For this review, take the finished solid that the model builds, in its own axes (mm). A direction names the side the tool comes from. Coordinates: 2 decimals unless noted, no trailing zeros. Loops run counter-clockwise (first coordinate to the right, second up) from the corner with the lowest first, then second, coordinate; pieces in that order, holes last. Notation, with made-up numbers: M -3,53.5 L 12,53.5 A30 ccw 12,77.5 Z; hole C 76.5,22 d4. An arc over 180 degrees is marked long. Use one line per item in the form item = value.
```python
from build123d import *

# Parameters (mm, degrees)
SKETCH1_W           = 69.85
SKETCH1_H           = 38.1
BOSS_EXTRUDE1_DEPTH = 3.175
SKETCH2_W           = 3.175
SKETCH2_H           = 3.175
BOSS_EXTRUDE2_DEPTH = 3.175
SKETCH3_W           = 20.32
SKETCH3_H           = 3.175
BOSS_EXTRUDE3_DEPTH = 3.175


with BuildPart() as part:
    # Sketch1 → Boss-Extrude1 (new body)
    with BuildSketch(Plane.XY):
        Rectangle(SKETCH1_W, SKETCH1_H)
    extrude(amount=BOSS_EXTRUDE1_DEPTH)

    # Sketch2 → Boss-Extrude2 (add)
    with BuildSketch(Plane(origin=(0, 0, 0), x_dir=(-1, 0, 0), z_dir=(0, 0, -1))):
        with Locations((-36.5125, 17.4625)):
            Rectangle(SKETCH2_W, SKETCH2_H)
        with Locations((-36.5125, -4.7625)):
            Rectangle(SKETCH2_W, SKETCH2_H)
        with Locations((36.5125, 17.4625)):
            Rectangle(SKETCH2_W, SKETCH2_H)
        with Locations((36.5125, -4.7625)):
            Rectangle(SKETCH2_W, SKETCH2_H)
    extrude(amount=-BOSS_EXTRUDE2_DEPTH)

    # Sketch3 → Boss-Extrude3 (add)
    with BuildSketch(Plane.XZ.offset(19.05)):
        with Locations((-16.51, 1.5875)):
            Rectangle(SKETCH3_W, SKETCH3_H)
        with Locations((16.51, 1.5875)):
            Rectangle(SKETCH3_W, SKETCH3_H)
    extrude(amount=BOSS_EXTRUDE3_DEPTH)


solid = part.part
```
1. Consider section C-C on x = 0. Write out the cut boundary in (y, z) (3 decimals).
Computed values:
outline = M -19.05,0 L 19.05,0 L 19.05,3.175 L -19.05,3.175 Z
2. Wall thickness on line 1 along X through (y, z) = (-20, 2.15); line 2 along X through (y, z) = (-13.5, 1.1) (3 decimals); line 3 along Y through (x, z) = (29, 1.95): over which ranges is each line inside the solid? List them lowest first. Write a range as from..to.
Computed values:
line_1 = -26.67..-6.35, 6.35..26.67
line_2 = -34.925..34.925
line_3 = -19.05..19.05
3. Draft analysis for pull direction Y (two halves, no side actions). For faces 6 (the face through (-36, -6.35, 2)), 7 (the face through (-38.1, -5, 2)), 8 (the face through (-36, 15.875, 2)), state which applies: +Y half, -Y half, draft (parallel to the pull), parting line (faces both ways), or undercut.
Computed values:
face_6 = -Y half
face_7 = draft
face_8 = undercut
4. Consider section A-A on z = 2.4. Write out the cut boundary in (x, y) (3 decimals).
Computed values:
outline = M -38.1,-6.35 L -34.925,-6.35 L -34.925,-19.05 L -26.67,-19.05 L -26.67,-22.225 L -6.35,-22.225 L -6.35,-19.05 L 6.35,-19.05 L 6.35,-22.225 L 26.67,-22.225 L 26.67,-19.05 L 34.925,-19.05 L 34.925,-6.35 L 38.1,-6.35 L 38.1,-3.175 L 34.925,-3.175 L 34.925,15.875 L 38.1,15.875 L 38.1,19.05 L -38.1,19.05 L -38.1,15.875 L -34.925,15.875 L -34.925,-3.175 L -38.1,-3.175 Z
5. For pin 1 Ø1.6 at (y, z) = (-10, 1.5) entering from -X (3 decimals); pin 2 Ø1 at (y, z) = (-11, 1) entering from +X (3 decimals); pin 3 Ø1.6 at (x, z) = (36, 2) entering from -Y, all flat-tipped, find the tip position at first contact; note any pin that passes through.
Computed values:
pin_1 = -34.925
pin_2 = 34.925
pin_3 = -6.35
6. Tool access review of faces 1 (the face through (-36, -3.175, 2)), 2 (the face through (34.925, -13, 2)), 3 (the face through (37, 15.875, 2)), 4 (the face through (-34.925, -13, 2)), 5 (the face through (-6.35, -21, 2)): name each direction out of +Z, -Z, +X, -X, +Y, -Y from which nothing blocks a thin tool from reaching the whole face with its end or side.
Computed values:
face_1 = +Z, -Z, -X
face_2 = +Z, -Z, +X, -Y
face_3 = +Z, -Z, +X
face_4 = +Z, -Z, -X, -Y
face_5 = +Z, -Z, -Y
7. Consider section B-B on y = -11. Write out the cut boundary in (x, z) (3 decimals), plus the area to 3 significant figures.
Computed values:
outline = M -34.925,0 L 34.925,0 L 34.925,3.175 L -34.925,3.175 Z
area = 222 mm2
